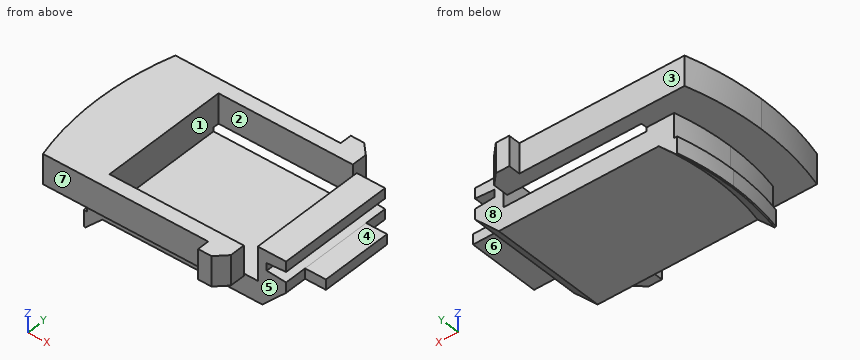
```python
from build123d import *

# Parameters (mm, degrees)
F1_DEPTH  = 4.6482
F2_SIZE   = 2.032
F3_W      = 12.192
F3_H      = 2.8702
F4_DEPTH  = 4.9794
F6_DEPTH  = 1.397
F7_SIZE   = 1.39699
F9_DEPTH  = 4.9794
F10_W     = 3.0734
F10_H     = 0.8720666667
F11_DEPTH = 1.778
F13_DEPTH = 2.54
F14_SIZE  = 0.889


# Not quite as in the source:
# - a fillet or chamfer is up to 0.001 mm smaller than in the source, because OpenCascade refuses the exact size


with BuildPart() as f1:
    # F0 (on Top) → F1 (new body)
    with BuildSketch(Plane.XY):
        with BuildLine():
            Line((-21.8694, 0), (-4.3434, 0))
            Line((-4.3434, 0), (-4.3434, 4.9784))
            Line((-4.3434, 4.9784), (-21.2952151856, 4.9784))
            ThreePointArc((-21.2952151856, 4.9784), (-21.7253795748, 2.5057012372), (-21.8694, 0))
        make_face()
    extrude(amount=F1_DEPTH)

    # F2
    f2_edges = [f1.edges().sort_by_distance(p)[0] for p in [
        (-4.3434, 2.4892, 0),
    ]]
    chamfer(f2_edges, length=F2_SIZE)

    # F3 (on face) → F4 (cut, through all)
    with BuildSketch(Plane.XZ):
        with Locations((-12.8524, 3.2131)):
            Rectangle(F3_W, F3_H)
    extrude(amount=-F4_DEPTH, mode=Mode.SUBTRACT)

    # F5 (on face) → F6 (join)
    with BuildSketch(Plane(origin=(0, 0, 0), x_dir=(1, 0, 0), z_dir=(0, 0, -1))):
        with BuildLine():
            ThreePointArc((-22.1234, 0), (-21.9810877831, -2.5053158344), (-21.5559820236, -4.9784))
            Line((-21.5559820236, -4.9784), (-19.9887671906, -4.9784))
            ThreePointArc((-19.9887671906, -4.9784), (-20.4461719061, -2.5078546104), (-20.5994, 0))
            Line((-20.5994, 0), (-22.1234, 0))
        make_face()
    extrude(amount=F6_DEPTH)

    # F7 (size 1.397 in the source; OpenCascade refuses exactly that, so slightly less here)
    f7_edges = [f1.edges().sort_by_distance(p)[0] for p in [
        (-20.446172, 2.507855, -1.397),
    ]]
    chamfer(f7_edges, length=F7_SIZE)

    # F8 (on face) → F9 (cut, through all)
    with BuildSketch(Plane.XZ):
        Polygon((-4.3434, 2.9040666667), (-4.3434, 3.7761333333), (-5.9944, 3.6576), (-5.9944, 3.0226), align=None)
    extrude(amount=-F9_DEPTH, mode=Mode.SUBTRACT)

    # F10 (on face) → F11 (join)
    with BuildSketch(Plane.YZ.offset(-4.3434)):
        with Locations((1.5367, 2.4680333333)):
            Rectangle(F10_W, F10_H)
    extrude(amount=F11_DEPTH)

    # F12 (on face) → F13 (join)
    with BuildSketch(Plane.XY.offset(4.6482)):
        with BuildLine():
            Line((-24.5364, 0), (-18.9484, 0))
            Line((-18.9484, 0), (-18.9484, 5.4864))
            Line((-18.9484, 5.4864), (-7.5184, 5.4864))
            Line((-7.5184, 5.4864), (-7.5184, 7.6835))
            Line((-7.5184, 7.6835), (-9.5504, 7.6835))
            Line((-9.5504, 7.6835), (-9.5504, 6.6675))
            Line((-9.5504, 6.6675), (-23.6131185723, 6.6675))
            ThreePointArc((-23.6131185723, 6.6675), (-24.3044836141, 3.3655610544), (-24.5364, 0))
        make_face()
    extrude(amount=-F13_DEPTH)

    # F14
    f14_edges = [f1.edges().sort_by_distance(p)[0] for p in [
        (-7.5184, 7.6835, 3.3782),
    ]]
    chamfer(f14_edges, length=F14_SIZE)

    # F15: F1 across face


with BuildPart() as f1_1:
    add(f1.part)
    add(f1.part.mirror(Plane(origin=(-14.9823216408, 0, 1.8516826104), x_dir=(1, 0, 0), z_dir=(0, -1, 0))))


solid = f1_1.part
```
Geometry check sheet. Reference: the model listing, model coordinates, mm. Face numbers are marked on the shaded views. A direction names the side the tool comes from. Give positions to 0.01 mm unless a question says otherwise; leave off trailing zeros. Write each loop counter-clockwise with the first axis right and the second up, starting at its lowest first coordinate (ties: lowest second). Pieces come first, ordered by that corner, then holes.
1) Gauge pin test, flat ends, axial feed: pin 1 (0.7 mm diameter, centred on y = -6, z = 4, fed in from +X); pin 2 (0.7 mm diameter, centred on y = -4.5, z = 2.5, fed in from +X); pin 3 (1.5 mm diameter, centred on x = -15, y = -0.5, fed in from +Z). Record the tip position at first contact, or that the pin passes through.
2) Section check A-A, the plane x = -17.75. Record the boundary of the cut face in (y, z), and give its area (3 significant figures).
3) Material ranges on L1, parallel to Z at x = -7.5, y = 0.75; L2, parallel to Y at x = -6, z = 2.5; L3, parallel to Y at x = -10, z = 4.25, recorded low to high.
4) Section check C-C, the plane x = -5. Record the boundary of the cut face in (y, z).
5) Section check D-D, the plane x = -9. Record the boundary of the cut face in (y, z).
6) Release check for a two-part mould opening along Y. For the marked faces 1, 2, 3 and 4 record: pulls with the +Y half, pulls with the -Y half, needs draft (parallel to the pull), parting line crosses it, or undercut.
7) Section check B-B, the plane z = 3.25. Record the boundary of the cut face in (x, y).
8) Access from +Z, -Z, +X, -X, +Y, -Y to the whole of each face (thin tool, end or side, straight path). Record for the marked faces 5, 6, 7 and 8.
Computed:
1. pin 1: stops at x = -7.52
1. pin 2: stops at x = -4.34
1. pin 3: stops at z = 1.78
2. outline: (-6.67, 2.11) - (-5.49, 2.11) - (-5.49, 4.65) - (-6.67, 4.65) - close; (-4.98, 0) - (4.98, 0) - (4.98, 1.78) - (-4.98, 1.78) - close; (5.49, 2.11) - (6.67, 2.11) - (6.67, 4.65) - (5.49, 4.65) - close
2. area: 23.7 mm2
3. L1: z = 0 to 1.78
3. L2: y = -4.98 to 4.98
3. L3: y = -6.67 to -5.49, 5.49 to 6.67
4. outline: (-4.98, 1.38) - (4.98, 1.38) - (4.98, 2.95) - (-4.98, 2.95) - close; (-4.98, 3.73) - (4.98, 3.73) - (4.98, 4.65) - (-4.98, 4.65) - close
5. outline: (-7.68, 2.11) - (-5.49, 2.11) - (-5.49, 4.65) - (-7.68, 4.65) - close; (-4.98, 0) - (4.98, 0) - (4.98, 1.78) - (-4.98, 1.78) - close; (5.49, 2.11) - (7.68, 2.11) - (7.68, 4.65) - (5.49, 4.65) - close
6. face 1: undercut
6. face 2: undercut
6. face 3: pulls with the +Y half
6. face 4: needs draft
7. outline: (-23.61, -6.67) - (-9.55, -6.67) - (-9.55, -7.68) - (-8.41, -7.68) - (-7.52, -6.79) - (-7.52, -5.49) - (-18.95, -5.49) - (-18.95, 5.49) - (-7.52, 5.49) - (-7.52, 6.79) - (-8.41, 7.68) - (-9.55, 7.68) - (-9.55, 6.67) - (-23.61, 6.67) arc R24.54 ccw to start; (-6.76, -4.98) - (-5.99, -4.98) - (-5.99, 4.98) - (-6.76, 4.98) - close
8. face 5: -Z, +X, -Y
8. face 6: -Z, +X, +Y, -Y
8. face 7: +Z, -Z, -X, -Y
8. face 8: -Z, +X, +Y
